Here's how the part is built. I have some questions about the finished solid (model axes, mm). Face numbers are marked on the shaded views. A direction names the side the tool comes from. Coordinates: 2 decimals unless noted, no trailing zeros. Write each loop counter-clockwise with the first axis right and the second up, starting at its lowest first coordinate (ties: lowest second). Pieces come first, ordered by that corner, then holes. Notation, with made-up numbers: M -29,-20.75 L 5,-20.75 A7 cw 5,-16.75 Z; hole C 38,-38.75 d2. An arc over 180 degrees is marked long. Use one line per item in the form item = value. Start each with the question number.
1. Thinking about a two-plate mould opening in Y: for the marked faces 1, 2 and 3, which applies, released by +Y, released by -Y, zero draft, split by the parting line, or undercut?
2. I want a section at B-B, the plane z = -11. Count the separate pieces of the cut face and the enclosed holes in it, plus the area to 3 significant figures.
3. On a 3-axis mill with a long thin cutter (end or side, diameter ignored), from which of +Z, -Z, +X, -X, +Y, -Y can I reach the whole of each face in a straight line? I mean the marked faces 4 and 5. Say none if no direction works.
4. I'm going to push flat-ended pins straight in: pin 1 Ø3 at (x, y) = (-38.89, 0) entering from -Z; pin 2 Ø6 at (x, y) = (11, 5.5) entering from -Z. Where does each tip first touch, or does it pass through?
5. I want a section at C-C, the plane x = -22. List the corners of the cut face in (y, z) for me (3 decimals).
6. I want a section at A-A, the plane y = 0. List the corners of the cut face in (x, z) for me (3 decimals).
7. Please list where these lines run through material, in increasing order: line 1 along X through (y, z) = (0.25, 1.75); line 2 along Y through (x, z) = (-34.5, -11.25) (3 decimals); line 3 along Y through (x, z) = (18.5, -8) (3 decimals). Write a range as [from, to].
from build123d import *

# Parameters (mm, degrees)
F1_W     = 88.9
F1_H     = 29.21
F2_DEPTH = 3.175
F3_W     = 88.9
F3_H     = 3.175
F4_DEPTH = 12.7
F6_D     = 3.3
F8_DEPTH = 3.175
F9_R     = 6.35
F10_R    = 3.175


# Not quite as in the source:
# - a variable given as a bare number and used for a length is read in inches; the dataset says mm whatever the document's units were


with BuildPart() as f2:
    # F1 (on Top) → F2 (new body)
    with BuildSketch(Plane.XY):
        Rectangle(F1_W, F1_H)
    extrude(amount=F2_DEPTH)

    # F3 (on face) → F4 (join)
    with BuildSketch(Plane(origin=(0, 0, 0), x_dir=(1, 0, 0), z_dir=(0, 0, -1))):
        with Locations((0, 13.0175)):
            Rectangle(F3_W, F3_H)
        with Locations((0, -13.0175)):
            Rectangle(F3_W, F3_H)
    extrude(amount=F4_DEPTH)

    # F6 (through all)
    with Locations(Plane.XY.offset(3.175)):
        with Locations((-38.89375, 0), (38.89375, 0)):
            Hole(F6_D / 2)

    # F7 (on face) → F8 (cut)
    with BuildSketch(Plane.XZ.offset(14.605)):
        with BuildLine():
            Line((-31.353125, -8.636), (-24.209375, -8.636))
            ThreePointArc((-24.209375, -8.636), (-27.78125, -5.064125), (-31.353125, -8.636))
        make_face()
        with BuildLine():
            Line((-24.209375, -12.7), (-24.209375, -8.636))
            ThreePointArc((-24.209375, -8.636), (-27.78125, -12.207875), (-31.353125, -8.636))
            Line((-31.353125, -8.636), (-31.353125, -12.7))
            Line((-31.353125, -12.7), (-24.209375, -12.7))
        make_face()
        with BuildLine():
            ThreePointArc((-31.353125, -8.636), (-27.78125, -12.207875), (-24.209375, -8.636))
            Line((-24.209375, -8.636), (-31.353125, -8.636))
        make_face()
        with BuildLine():
            Line((-20.240625, -8.636), (-13.096875, -8.636))
            ThreePointArc((-13.096875, -8.636), (-16.66875, -5.064125), (-20.240625, -8.636))
        make_face()
        with BuildLine():
            Line((-13.096875, -12.7), (-13.096875, -8.636))
            ThreePointArc((-13.096875, -8.636), (-16.66875, -12.207875), (-20.240625, -8.636))
            Line((-20.240625, -8.636), (-20.240625, -12.7))
            Line((-20.240625, -12.7), (-13.096875, -12.7))
        make_face()
        with BuildLine():
            ThreePointArc((-20.240625, -8.636), (-16.66875, -12.207875), (-13.096875, -8.636))
            Line((-13.096875, -8.636), (-20.240625, -8.636))
        make_face()
        with BuildLine():
            Line((-9.128125, -8.636), (-1.984375, -8.636))
            ThreePointArc((-1.984375, -8.636), (-5.55625, -5.064125), (-9.128125, -8.636))
        make_face()
        with BuildLine():
            Line((-1.984375, -12.7), (-1.984375, -8.636))
            ThreePointArc((-1.984375, -8.636), (-5.55625, -12.207875), (-9.128125, -8.636))
            Line((-9.128125, -8.636), (-9.128125, -12.7))
            Line((-9.128125, -12.7), (-1.984375, -12.7))
        make_face()
        with BuildLine():
            ThreePointArc((-9.128125, -8.636), (-5.55625, -12.207875), (-1.984375, -8.636))
            Line((-1.984375, -8.636), (-9.128125, -8.636))
        make_face()
        with BuildLine():
            Line((1.984375, -8.636), (9.128125, -8.636))
            ThreePointArc((9.128125, -8.636), (5.55625, -5.064125), (1.984375, -8.636))
        make_face()
        with BuildLine():
            Line((9.128125, -12.7), (9.128125, -8.636))
            ThreePointArc((9.128125, -8.636), (5.55625, -12.207875), (1.984375, -8.636))
            Line((1.984375, -8.636), (1.984375, -12.7))
            Line((1.984375, -12.7), (9.128125, -12.7))
        make_face()
        with BuildLine():
            ThreePointArc((1.984375, -8.636), (5.55625, -12.207875), (9.128125, -8.636))
            Line((9.128125, -8.636), (1.984375, -8.636))
        make_face()
        with BuildLine():
            Line((13.096875, -8.636), (20.240625, -8.636))
            ThreePointArc((20.240625, -8.636), (16.66875, -5.064125), (13.096875, -8.636))
        make_face()
        with BuildLine():
            Line((20.240625, -12.7), (20.240625, -8.636))
            ThreePointArc((20.240625, -8.636), (16.66875, -12.207875), (13.096875, -8.636))
            Line((13.096875, -8.636), (13.096875, -12.7))
            Line((13.096875, -12.7), (20.240625, -12.7))
        make_face()
        with BuildLine():
            ThreePointArc((13.096875, -8.636), (16.66875, -12.207875), (20.240625, -8.636))
            Line((20.240625, -8.636), (13.096875, -8.636))
        make_face()
        with BuildLine():
            Line((24.209375, -8.636), (31.353125, -8.636))
            ThreePointArc((31.353125, -8.636), (27.78125, -5.064125), (24.209375, -8.636))
        make_face()
        with BuildLine():
            Line((31.353125, -12.7), (31.353125, -8.636))
            ThreePointArc((31.353125, -8.636), (27.78125, -12.207875), (24.209375, -8.636))
            Line((24.209375, -8.636), (24.209375, -12.7))
            Line((24.209375, -12.7), (31.353125, -12.7))
        make_face()
        with BuildLine():
            ThreePointArc((24.209375, -8.636), (27.78125, -12.207875), (31.353125, -8.636))
            Line((31.353125, -8.636), (24.209375, -8.636))
        make_face()
    extrude(amount=-F8_DEPTH, mode=Mode.SUBTRACT)

    # F9
    f9_edges = [f2.edges().sort_by_distance(p)[0] for p in [
        (0, -14.605, 3.175),
        (0, 14.605, 3.175),
    ]]
    fillet(f9_edges, radius=F9_R)

    # F10
    f10_edges = [f2.edges().sort_by_distance(p)[0] for p in [
        (0, 11.43, 0),
        (0, -11.43, 0),
    ]]
    fillet(f10_edges, radius=F10_R)


solid = f2.part
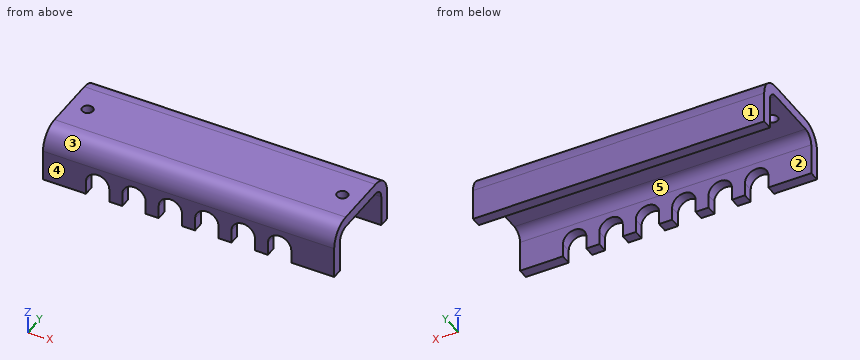
Answer list:
q1.face_1 = released by +Y
q1.face_2 = undercut
q1.face_3 = released by -Y
q2.separate_pieces = 8
q2.enclosed_holes = 0
q2.area = 428 mm²
q3.face_4 = +Z, -Z, +X, -X, -Y
q3.face_5 = -Z, +X, -X
q4.pin_1 = through
q4.pin_2 = -0.01
q5.outline = M -14.605,-12.7 L -11.43,-12.7 L -11.43,-3.175 A3.175 cw -8.255,0 L 8.255,0 A3.175 cw 11.43,-3.175 L 11.43,-12.7 L 14.605,-12.7 L 14.605,-3.175 A6.35 ccw 8.255,3.175 L -8.255,3.175 A6.35 ccw -14.605,-3.175 Z
q6.outline = M -44.45,0 L -40.544,0 L -40.544,3.175 L -44.45,3.175 Z; M -37.244,0 L 37.244,0 L 37.244,3.175 L -37.244,3.175 Z; M 40.544,0 L 44.45,0 L 44.45,3.175 L 40.544,3.175 Z
q7.line_1 = [-44.45, -40.52], [-37.26, 37.26], [40.52, 44.45]
q7.line_2 = [-14.605, -11.43], [11.43, 14.605]
q7.line_3 = [11.43, 14.605]
